Here's how the part is built. I have some questions about the finished solid (model axes, mm). A direction names the side the tool comes from. Round coordinates to 2 decimals unless told otherwise and drop trailing zeros. Order: outer loops, then holes, each group sorted by start corner. A loop starts at its lowest first (then second) coordinate and runs counter-clockwise, first axis right, second up.
Autodesk Inventor part; units mm, degrees
ref_plane "YZ Plane" through (0, 0, 0) normal (1, 0, 0) x (0, 1, 0)
ref_plane "XZ Plane" through (0, 0, 0) normal (0, 1, 0) x (-1, 0, 0)
ref_plane "XY Plane" through (0, 0, 0) normal (0, 0, 1) x (1, 0, 0)
sketch "Sketch1" plane through (0, 0, 0) normal (1, 0, 0) x (0, 1, 0)
  line L0 (0, 0) -> (50.8, 0)
  line L1 (50.8, 0) -> (50.8, -177.8)
  line L2 (50.8, -177.8) -> (0, -177.8)
  line L3 (0, -177.8) -> (0, 0)
  dimension "d0" = 50.8
  dimension "d1" = 177.8
extrude "Extrusion1" add sketch "Sketch1" along normal blind 25.4
shell "Shell1" thickness 3.175 removed faces 2 at (8.4667, 16.9333, 0) at (8.4667, 33.8667, -177.8)
sketch "Sketch2" plane through (25.4, 0, 0) normal (1, 0, 0) x (0, 0, -1)
  line L0 (0, 3.175) -> (0, 47.625) construction
  line L1 (0, 25.4) -> (177.8, 25.4) construction
  line L2 (177.8, 3.175) -> (177.8, 47.625) construction
  line L3 (0, 25.4) -> (25.4, 25.4) construction
  circle A0 centre (25.4, 25.4) radius 14.2875
  line L4 (25.4, 25.4) -> (76.2, 25.4) construction
  circle A1 centre (76.2, 25.4) radius 14.2875
  circle A2 centre (25.4, 25.4) radius 19.05 construction
  circle A3 centre (76.2, 25.4) radius 19.05 construction
  line L5 (177.8, 50.8) -> (0, 50.8) construction
  line L6 (0, 50.8) -> (12.7, 50.8) construction
  line L7 (12.7, 50.8) -> (12.7, 38.1) construction
  line L8 (12.7, 38.1) -> (0, 38.1) construction
  line L9 (0, 38.1) -> (0, 50.8) construction
  line L10 (0, 0) -> (12.7, 0) construction
  line L11 (12.7, 0) -> (12.7, 12.7) construction
  line L12 (12.7, 12.7) -> (0, 12.7) construction
  line L13 (0, 12.7) -> (0, 0) construction
  line L14 (177.8, 50.8) -> (165.1, 50.8) construction
  line L15 (165.1, 50.8) -> (165.1, 38.1) construction
  line L16 (165.1, 38.1) -> (177.8, 38.1) construction
  line L17 (177.8, 38.1) -> (177.8, 50.8) construction
  line L18 (177.8, 0) -> (165.1, 0) construction
  line L19 (165.1, 0) -> (165.1, 12.7) construction
  line L20 (165.1, 12.7) -> (177.8, 12.7) construction
  line L21 (177.8, 12.7) -> (177.8, 0) construction
  line L22 (177.8, 50.8) -> (139.7, 50.8) construction
  line L23 (139.7, 50.8) -> (139.7, 38.1) construction
  line L24 (139.7, 38.1) -> (177.8, 38.1) construction
  line L25 (177.8, 38.1) -> (177.8, 50.8) construction
  line L26 (177.8, 0) -> (139.7, 0) construction
  line L27 (139.7, 0) -> (139.7, 12.7) construction
  line L28 (139.7, 12.7) -> (177.8, 12.7) construction
  line L29 (177.8, 12.7) -> (177.8, 0) construction
  circle A4 centre (165.1, 12.7) radius 2.5797
  circle A5 centre (139.7, 12.7) radius 2.5797
  dimension "d5" = 25.4
  dimension "d6" = 28.575
  dimension "d7" = 50.8
  dimension "d8" = 28.575
  dimension "d9" = 38.1
  dimension "d10" = 38.1
  dimension "d11" = 12.7
  dimension "d12" = 12.7
  dimension "d13" = 12.7
  dimension "d14" = 12.7
  dimension "d15" = 12.7
  dimension "d16" = 12.7
  dimension "d17" = 12.7
  dimension "d18" = 12.7
  dimension "d19" = 38.1
  dimension "d20" = 38.1
  dimension "d22" = 5.1594
  dimension "d23" = 5.1594
extrude "Extrusion2" cut sketch "Sketch2" against normal blind 50.8
hole "Hole1" at (12.7, 0, -12.7) direction (0, 1, 0) diameter 5.1594 end through all
hole "Hole2" at (12.7, 0, -38.1) direction (0, 1, 0) diameter 5.1594 end through all
properties part number "Top Roller Wheel Mount"
1. If we section it at A-A, the plane x = 8.5: Write out the boundary of the cut face in (y, z) (3 decimals).
Evaluation:
outline: (0, -177.8) - (3.175, -177.8) - (3.175, 0) - (0, 0) - close; (47.625, -177.8) - (50.8, -177.8) - (50.8, 0) - (47.625, 0) - close
2. If we section it at D-D, the plane y = 25.4: Write out the boundary of the cut face in (x, z) (1 decimal), and give its area (3 significant figures).
Evaluation:
outline: (0, -177.8) - (3.2, -177.8) - (3.2, -90.5) - (0, -90.5) - close; (0, -61.9) - (3.2, -61.9) - (3.2, -39.7) - (0, -39.7) - close; (0, -11.1) - (3.2, -11.1) - (3.2, 0) - (0, 0) - close; (22.2, -177.8) - (25.4, -177.8) - (25.4, -90.5) - (22.2, -90.5) - close; (22.2, -61.9) - (25.4, -61.9) - (25.4, -39.7) - (22.2, -39.7) - close; (22.2, -11.1) - (25.4, -11.1) - (25.4, 0) - (22.2, 0) - close
area: 766 mm2
3. If we section it at C-C, the plane y = 44.5: Write out the boundary of the cut face in (x, z) (3 decimals), and give its area (3 significant figures).
Evaluation:
outline: (0, -177.8) - (3.175, -177.8) - (3.175, 0) - (0, 0) - close; (22.225, -177.8) - (25.4, -177.8) - (25.4, 0) - (22.225, 0) - close
area: 1,130 mm2
4. If we mould it in two halves opening along X, with no side actions, what happens to faces 1 (the flat face through (25.4, 36, -88)), 2 (the cylindrical face through (10.525, 1.61, -14.087)), 3 (the flat face through (13, 50.8, -88))? For each: released by +X, released by -X, zero draft, split by the parting line, or undercut.
Evaluation:
face 1: released by +X
face 2: undercut
face 3: zero draft
5. On a 3-axis mill with a long thin cutter (end or side, diameter ignored), from which of +Z, -Z, +X, -X, +Y, -Y can I reach the whole of each face in a straight line? I mean faces 4 (the flat face through (22.225, 35, -88)), 5 (the cylindrical face through (11.925, 49.235, -40.561)). Say none if no direction works.
Evaluation:
face 4: +Z, -Z
face 5: +Y, -Y
6. I need wall thicknesses on probe 1 along Z at (x, y) = (12.7, 2); probe 2 along Y at (x, z) = (4.5, -39) (3 decimals); probe 3 along Y at (x, z) = (23.9, -165.1). Which ranges of each line are inside material? Lowest first, please.
Evaluation:
probe 1: z = -177.8 to -40.68, -35.52 to -15.28, -10.12 to 0
probe 2: y = 0 to 3.175, 47.625 to 50.8
probe 3: y = 0 to 10.12, 15.28 to 50.8
7. If we section it at B-B, the plane z = -165.1: Write out the boundary of the cut face in (x, y) (3 decimals), and give its area (3 significant figures).
Evaluation:
outline: (0, 0) - (25.4, 0) - (25.4, 10.12) - (22.225, 10.12) - (22.225, 3.175) - (3.175, 3.175) - (3.175, 10.12) - (0, 10.12) - close; (0, 15.28) - (3.175, 15.28) - (3.175, 47.625) - (22.225, 47.625) - (22.225, 15.28) - (25.4, 15.28) - (25.4, 50.8) - (0, 50.8) - close
area: 411 mm2
